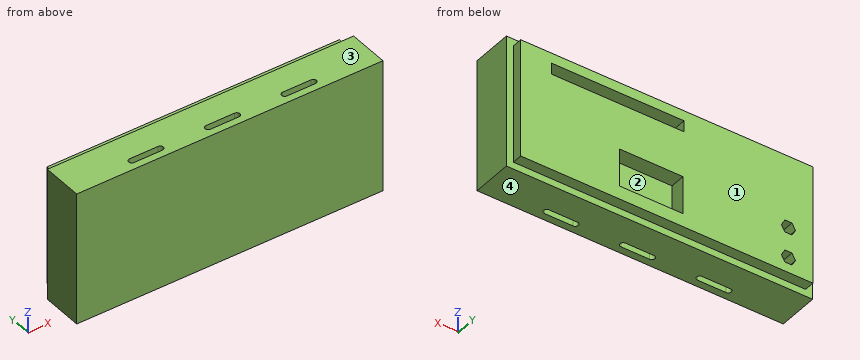
from build123d import *

# Parameters (mm, degrees)
SKETCH1_W           = 150
SKETCH1_H           = 65
BOSS_EXTRUDE1_DEPTH = 20
CUT_EXTRUDE1_DEPTH  = 66
SKETCH3_W           = 143.142
SKETCH3_H           = 58.142
BOSS_EXTRUDE2_DEPTH = 5
CUT_EXTRUDE2_DEPTH  = 6.5
SKETCH6_W           = 65
SKETCH6_H           = 5.5
CUT_EXTRUDE3_DEPTH  = 10
SKETCH7_W           = 31
SKETCH7_H           = 18.5
CUT_EXTRUDE4_DEPTH  = 7.5


with BuildPart() as part:
    # Sketch1 → Boss-Extrude1 (new body)
    with BuildSketch(Plane(origin=(0, 0, 0), x_dir=(1, 0, 0), z_dir=(0, 1, 0))):
        Rectangle(SKETCH1_W, SKETCH1_H)
    extrude(amount=BOSS_EXTRUDE1_DEPTH)

    # Sketch2 → Cut-Extrude1 (cut, through all)
    with BuildSketch(Plane.XY.offset(32.5)):
        with BuildLine():
            Line((-7, 6.5), (7, 6.5))
            ThreePointArc((7, 6.5), (8.5, 5), (7, 3.5))
            Line((7, 3.5), (-7, 3.5))
            ThreePointArc((-7, 3.5), (-8.5, 5), (-7, 6.5))
        make_face()
        with BuildLine():
            Line((-44.5, 6.5), (-30.5, 6.5))
            ThreePointArc((-30.5, 6.5), (-29, 5), (-30.5, 3.5))
            Line((-30.5, 3.5), (-44.5, 3.5))
            ThreePointArc((-44.5, 3.5), (-46, 5), (-44.5, 6.5))
        make_face()
        with BuildLine():
            Line((30.5, 6.5), (44.5, 6.5))
            ThreePointArc((44.5, 6.5), (46, 5), (44.5, 3.5))
            Line((44.5, 3.5), (30.5, 3.5))
            ThreePointArc((30.5, 3.5), (29, 5), (30.5, 6.5))
        make_face()
    extrude(amount=-CUT_EXTRUDE1_DEPTH, mode=Mode.SUBTRACT)

    # Sketch3 → Boss-Extrude2 (add)
    with BuildSketch(Plane(origin=(0, 20, 0), x_dir=(1, 0, 0), z_dir=(0, 1, 0))):
        Rectangle(SKETCH3_W, SKETCH3_H)
    extrude(amount=BOSS_EXTRUDE2_DEPTH)

    # Sketch4 → Cut-Extrude2 (cut)
    with BuildSketch(Plane(origin=(0, 25, 0), x_dir=(1, 0, 0), z_dir=(0, 1, 0))):
        Polygon((-61.303050808, 24.571), (-63.035101615, 21.571), (-61.303050808, 18.571), (-57.838949192, 18.571), (-56.106898385, 21.571), (-57.838949192, 24.571), align=None)
        Polygon((-61.303050808, 9.551), (-63.035101615, 6.551), (-61.303050808, 3.551), (-57.838949192, 3.551), (-56.106898385, 6.551), (-57.838949192, 9.551), align=None)
    extrude(amount=-CUT_EXTRUDE2_DEPTH, mode=Mode.SUBTRACT)

    # Sketch6 → Cut-Extrude3 (cut)
    with BuildSketch(Plane(origin=(0, 25, 0), x_dir=(1, 0, 0), z_dir=(0, 1, 0))):
        with Locations((24.071, -21.321)):
            Rectangle(SKETCH6_W, SKETCH6_H)
    extrude(amount=-CUT_EXTRUDE3_DEPTH, mode=Mode.SUBTRACT)

    # Sketch7 → Cut-Extrude4 (cut)
    with BuildSketch(Plane(origin=(0, 25, 0), x_dir=(1, 0, 0), z_dir=(0, 1, 0))):
        with Locations((7.571, 13.321)):
            Rectangle(SKETCH7_W, SKETCH7_H)
    extrude(amount=-CUT_EXTRUDE4_DEPTH, mode=Mode.SUBTRACT)


solid = part.part
Source: CAD feature listing. Evaluate the final solid. Frame: model axes, mm. Face numbers are marked on the shaded views. Give positions to 0.01 mm unless a question says otherwise; leave off trailing zeros. Write each loop counter-clockwise with the first axis right and the second up, starting at its lowest first coordinate (ties: lowest second). Pieces come first, ordered by that corner, then holes. Notation, with made-up numbers: (2.25, 34.5) -> (17.25, 34.5) arc R24 cw to (17.25, 66.5) -> close; hole circle Ø8 at (18, 2). An arc over 180 degrees is marked (long way). Return JSON: item names as keys, results as strings. Group by question number.
1. Pin query (flat end, axial travel): pin 1 Ø1 at (x, y) = (-58.5, 22.5) entering from +Z; pin 2 Ø1.6 at (y, z) = (21.5, 21) entering from +X; pin 3 Ø3 at (x, z) = (16, 22) entering from +Y. Return the tip coordinate at first contact, or that it passes through.
2. Section D-D, the plane x = -51. Output: boundary loops of the cut face in (y, z).
3. Section B-B, the plane y = 5. Output: boundary loops of the cut face in (x, z), then the cut area to 4 significant figures.
4. Material intervals for line 1 (Y direction, x = 35, z = 15); line 2 (X direction, y = 4.25, z = 6.5); line 3 (X direction, y = 5.5, z = 8), sorted ascending. Write a range as from..to.
5. Mould query, pull axis Z, two halves, no side actions, for the marked faces 1, 2, 3 and 4. Classes: +Z half, -Z half, draft (parallel to the pull), parting line (faces both ways), or undercut.
6. Section A-A, the plane x = -35. Output: boundary loops of the cut face in (y, z), then the cut area to 3 significant figures.
7. Section C-C, the plane z = -0.5. Output: boundary loops of the cut face in (x, y), then the cut area to 3 significant figures.
Determined:
{
 "1": {"pin 1": "stops at z = 29.07", "pin 2": "stops at x = 71.57", "pin 3": "stops at y = 15"},
 "2": {"outline": "(0, -32.5) -> (20, -32.5) -> (20, -29.07) -> (25, -29.07) -> (25, 29.07) -> (20, 29.07) -> (20, 32.5) -> (0, 32.5) -> close"},
 "3": {"outline": "(-75, -32.5) -> (-46, -32.5) -> (-46, 32.5) -> (-75, 32.5) -> close; (-29, -32.5) -> (-8.5, -32.5) -> (-8.5, 32.5) -> (-29, 32.5) -> close; (8.5, -32.5) -> (29, -32.5) -> (29, 32.5) -> (8.5, 32.5) -> close; (46, -32.5) -> (75, -32.5) -> (75, 32.5) -> (46, 32.5) -> close", "area": "6,435 mm2"},
 "4": {"line 1": "y = 0..3.5, 6.5..25", "line 2": "x = -75..-45.8, -29.2..-8.3, 8.3..29.2, 45.8..75", "line 3": "x = -75..-45.91, -29.09..-8.41, 8.41..29.09, 45.91..75"},
 "5": {"face 1": "draft", "face 2": "undercut", "face 3": "+Z half", "face 4": "-Z half"},
 "6": {"outline": "(0, -32.5) -> (3.5, -32.5) -> (3.5, 32.5) -> (0, 32.5) -> close; (6.5, -32.5) -> (20, -32.5) -> (20, -29.07) -> (25, -29.07) -> (25, 29.07) -> (20, 29.07) -> (20, 32.5) -> (6.5, 32.5) -> close", "area": "1,400 mm2"},
 "7": {"outline": "(-75, 0) -> (75, 0) -> (75, 20) -> (71.57, 20) -> (71.57, 25) -> (-71.57, 25) -> (-71.57, 20) -> (-75, 20) -> close; hole (-44.5, 3.5) -> (-30.5, 3.5) arc R1.5 ccw to (-30.5, 6.5) -> (-44.5, 6.5) arc R1.5 ccw to start; hole (-7, 3.5) -> (7, 3.5) arc R1.5 ccw to (7, 6.5) -> (-7, 6.5) arc R1.5 ccw to start; hole (30.5, 3.5) -> (44.5, 3.5) arc R1.5 ccw to (44.5, 6.5) -> (30.5, 6.5) arc R1.5 ccw to start", "area": "3,570 mm2"}
}
